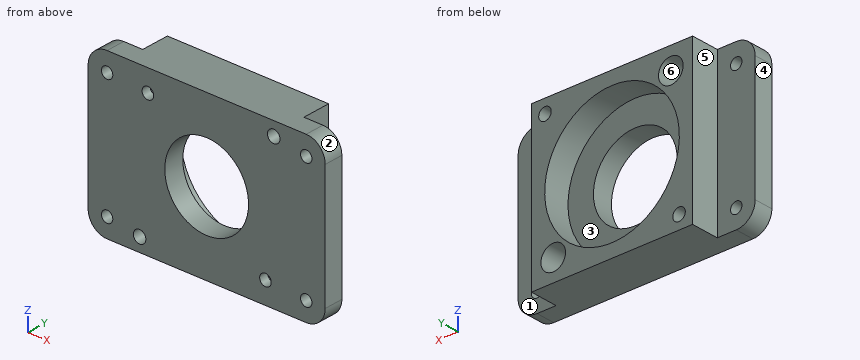
```python
from build123d import *

# Parameters (mm, degrees)
SKETCH_1_W          = 42.5
SKETCH_1_H          = 42.5
EXTRUDE_1_DEPTH     = 12.4
SKETCH_2_R          = 17.75
CUT_EXTRUDE_1_DEPTH = 7
SKETCH_3_R          = 11.05
CUT_EXTRUDE_2_DEPTH = 61.510329697
SKETCH_4_R          = 3.25
SKETCH_4_R_2        = 1.525
CUT_EXTRUDE_3_DEPTH = 10
SKETCH_4_3_R        = 1.525
SKETCH_4_3_R_2      = 1.65
CUT_EXTRUDE_4_DEPTH = 62.36986231
SKETCH_5_W          = 10
SKETCH_5_H          = 42.5
SKETCH_5_R          = 1.5
EXTRUDE_2_DEPTH     = 5
FILLET_1_R          = 5


with BuildPart() as part:
    # Sketch 1 → Extrude 1 (new body)
    with BuildSketch(Plane(origin=(0, 0, 0), x_dir=(1, 0, 0), z_dir=(0, 1, 0))):
        with Locations((21.25, 21.25)):
            Rectangle(SKETCH_1_W, SKETCH_1_H)
    extrude(amount=EXTRUDE_1_DEPTH)

    # Sketch 2 → Cut-Extrude 1 (cut)
    with BuildSketch(Plane(origin=(0, 12.4, 0), x_dir=(1, 0, 0), z_dir=(0, 1, 0))):
        with Locations(Location((21.25, 21.25, 0), (0, 0, 270))):
            Circle(SKETCH_2_R)
    extrude(amount=-CUT_EXTRUDE_1_DEPTH, mode=Mode.SUBTRACT)

    # Sketch 3 → Cut-Extrude 2 (cut, through all)
    with BuildSketch(Plane(origin=(0, 5.4, 0), x_dir=(1, 0, 0), z_dir=(0, 1, 0))):
        with Locations(Location((21.25, 21.25, 0), (0, 0, 270))):
            Circle(SKETCH_3_R)
    extrude(amount=-CUT_EXTRUDE_2_DEPTH, mode=Mode.SUBTRACT)

    # Sketch 4 → Cut-Extrude 3 (cut)
    # profile 1 of 4: a face of its own
    with BuildSketch(Plane(origin=(0, 12.4, 0), x_dir=(1, 0, 0), z_dir=(0, 1, 0))):
        with Locations(Location((5.75, 5.75, 0), (0, 0, 270))):
            Circle(SKETCH_4_R)
        with Locations((5.75, 5.75)):
            Circle(SKETCH_4_R_2, mode=Mode.SUBTRACT)
    # profile 2 of 4: a face of its own
    with BuildSketch(Plane(origin=(0, 12.4, 0), x_dir=(1, 0, 0), z_dir=(0, 1, 0))):
        with Locations((5.75, 5.75)):
            Circle(SKETCH_4_R_2)
    # profile 3 of 4: a face of its own
    with BuildSketch(Plane(origin=(0, 12.4, 0), x_dir=(1, 0, 0), z_dir=(0, 1, 0))):
        with Locations(Location((36.75, 36.75, 0), (0, 0, 270))):
            Circle(SKETCH_4_R)
        with Locations((36.75, 36.75)):
            Circle(SKETCH_4_R_2, mode=Mode.SUBTRACT)
    # profile 4 of 4: a face of its own
    with BuildSketch(Plane(origin=(0, 12.4, 0), x_dir=(1, 0, 0), z_dir=(0, 1, 0))):
        with Locations((36.75, 36.75)):
            Circle(SKETCH_4_R_2)
    extrude(amount=-CUT_EXTRUDE_3_DEPTH, mode=Mode.SUBTRACT)

    # Sketch 4_3 → Cut-Extrude 4 (cut, through all)
    with BuildSketch(Plane(origin=(0, 12.4, 0), x_dir=(1, 0, 0), z_dir=(0, 1, 0))):
        with Locations(Location((5.75, 5.75, 0), (0, 0, 270))):
            Circle(SKETCH_4_3_R)
        with Locations(Location((38.92766953, 3.57233047, 0), (0, 0, 270))):
            Circle(SKETCH_4_3_R_2)
        with Locations(Location((36.75, 36.75, 0), (0, 0, 270))):
            Circle(SKETCH_4_3_R)
        with Locations(Location((3.57233047, 38.92766953, 0), (0, 0, 270))):
            Circle(SKETCH_4_3_R_2)
    extrude(amount=-CUT_EXTRUDE_4_DEPTH, mode=Mode.SUBTRACT)

    # Sketch 5 → Extrude 2 (add)
    # profile 1 of 2: a face of its own
    with BuildSketch(Plane.XZ):
        with Locations((-5, -21.25)):
            Rectangle(SKETCH_5_W, SKETCH_5_H)
        with Locations(Location((-5, -5, 0), (0, 0, 270))):
            Circle(SKETCH_5_R, mode=Mode.SUBTRACT)
        with Locations(Location((-5, -37.5, 0), (0, 0, 270))):
            Circle(SKETCH_5_R, mode=Mode.SUBTRACT)
    # profile 2 of 2: a face of its own
    with BuildSketch(Plane.XZ):
        with Locations((47.5, -21.25)):
            Rectangle(SKETCH_5_W, SKETCH_5_H)
        with Locations(Location((47.5, -37.5, 0), (0, 0, 270))):
            Circle(SKETCH_5_R, mode=Mode.SUBTRACT)
        with Locations(Location((47.5, -5, 0), (0, 0, 270))):
            Circle(SKETCH_5_R, mode=Mode.SUBTRACT)
    extrude(amount=-EXTRUDE_2_DEPTH)

    # Fillet 1
    fillet_1_edges = [part.edges().sort_by_distance(p)[0] for p in [
        (-10, 2.5, -42.5),
        (-10, 2.5, 0),
        (52.5, 2.5, 0),
        (52.5, 2.5, -42.5),
    ]]
    fillet(fillet_1_edges, radius=FILLET_1_R)


solid = part.part
```
CAD build for the part. Positions are in the model's coordinates, mm. Face numbers are marked on the shaded views. A direction names the side the tool comes from. Round coordinates to 2 decimals unless told otherwise and drop trailing zeros. Order: outer loops, then holes, each group sorted by start corner. A loop starts at its lowest first (then second) coordinate and runs counter-clockwise, first axis right, second up.
Item 1: Saw through at A-A on x = 21.25. Write the cut outline in (y, z), then the cut area to 3 significant figures.
Item 2: Pin check, flat tips, straight feed: pin 1 (3 mm diameter, centred on x = 3.57, z = -38.93, fed in from +Y); pin 2 (5 mm diameter, centred on x = -6, z = -30, fed in from +Y). Stop position of each tip, or through.
Item 3: Saw through at D-D on x = 14. Write the cut outline in (y, z), then the cut area to 3 significant figures.
Item 4: Tool access for the marked faces 4, 5 and 6: list every direction of +Z, -Z, +X, -X, +Y, -Y with a clear straight run to the whole face (end or side of a thin tool).
Item 5: Probe line 1 along X through (y, z) = (10, -37.5); line 2 along X through (y, z) = (2.35, -37.5); line 3 along X through (y, z) = (9.25, -21.25). List the from-to ranges inside material, lowest first.
Item 6: Saw through at C-C on y = 3.5. State how many separate pieces and enclosed holes the cut face has, then the cut area to 3 significant figures.
Item 7: Mould opens along Z. For the marked faces 1, 2 and 3 say: pulls with the +Z half, pulls with the -Z half, needs draft (parallel to the pull), parting line crosses it, or undercut.
Item 8: Saw through at B-B on z = -21.25. Write the cut outline in (x, y), then the cut area to 3 significant figures.
Reported:
1. outline: (0, -42.5) - (12.4, -42.5) - (12.4, -39) - (5.4, -39) - (5.4, -32.3) - (0, -32.3) - close; (0, -10.2) - (5.4, -10.2) - (5.4, -3.5) - (12.4, -3.5) - (12.4, 0) - (0, 0) - close
1. area: 159 mm2
2. pin 1: passes through
2. pin 2: stops at y = 5
3. outline: (0, -42.5) - (12.4, -42.5) - (12.4, -37.45) - (5.4, -37.45) - (5.4, -29.59) - (0, -29.59) - close; (0, -12.91) - (5.4, -12.91) - (5.4, -5.05) - (12.4, -5.05) - (12.4, 0) - (0, 0) - close
3. area: 210 mm2
4. face 4: +Z, -Z, -X, +Y, -Y
4. face 5: +Z, -Z, -X, +Y
4. face 6: +Y
5. line 1: x = 0 to 2.75, 4.4 to 14.11, 28.39 to 33.59, 39.91 to 42.5
5. line 2: x = -10 to -6.5, -3.5 to 2.75, 4.4 to 35.42, 38.08 to 46, 49 to 52.5
5. line 3: x = 0 to 3.5, 39 to 42.5
6. separate pieces: 1
6. enclosed holes: 9
6. area: 2,140 mm2
7. face 1: needs draft
7. face 2: pulls with the +Z half
7. face 3: undercut
8. outline: (-10, 0) - (10.2, 0) - (10.2, 5.4) - (3.5, 5.4) - (3.5, 12.4) - (0, 12.4) - (0, 5) - (-10, 5) - close; (32.3, 0) - (52.5, 0) - (52.5, 5) - (42.5, 5) - (42.5, 12.4) - (39, 12.4) - (39, 5.4) - (32.3, 5.4) - close
8. area: 259 mm2
